```python
from build123d import *

# Parameters (mm, degrees)
CROQUIS1_R                 = 2
SALIENTE_EXTRUIR1_DEPTH    = 21
CORTAR_EXTRUIR1_DEPTH      = 43.09513036
CORTAR_EXTRUIR1_DEPTH_BACK = 5
CUT_EXTRUDE1_START         = 10
SKETCH2_R                  = 1.25
CUT_EXTRUDE1_DEPTH         = 3
LPATTERN1_COUNT            = 2
LPATTERN1_PITCH            = 20


with BuildPart() as part:
    # Croquis1 → Saliente-Extruir1 (new, symmetric)
    with BuildSketch(Plane(origin=(0, 0, 0), x_dir=(1, 0, 0), z_dir=(0, 1, 0))):
        with Locations(Location((0, 0, 0), (0, 0, 90))):
            Circle(CROQUIS1_R)
    extrude(amount=SALIENTE_EXTRUIR1_DEPTH, both=True)

    # Croquis2 → Cortar-Extruir1 (cut, two sides: drawn at the far end of the back side and taken through both)
    with BuildSketch(Plane(origin=(0, 21, 0), x_dir=(1, 0, 0), z_dir=(0, 1, 0)).offset(-CORTAR_EXTRUIR1_DEPTH_BACK)):
        Polygon((-21.233275663, 1.2), (-1.6, 1.2), (1.6, 1.2), (21.233275663, 1.2), (21.233275663, 40.466551326), (-21.233275663, 40.466551326), align=None)
    extrude(amount=CORTAR_EXTRUIR1_DEPTH + CORTAR_EXTRUIR1_DEPTH_BACK, mode=Mode.SUBTRACT)

    # Sketch2 → Cut-Extrude1 (cut)
    with BuildSketch(Plane(origin=(0, 0, 0), x_dir=(1, 0, 0), z_dir=(0, 1, 0)).offset(CUT_EXTRUDE1_START)):
        with Locations((2, 0)):
            Circle(SKETCH2_R)
    cut_extrude1 = extrude(amount=-CUT_EXTRUDE1_DEPTH, mode=Mode.SUBTRACT)

    # LPattern1: Cut-Extrude1 ×2
    with Locations(*[(0, -i * LPATTERN1_PITCH, 0) for i in range(1, LPATTERN1_COUNT)]):
        add(cut_extrude1, mode=Mode.SUBTRACT)


solid = part.part
```
Input: part model. Units: mm. Frame: model coordinates. A direction names the side the tool comes from. Give positions to 0.01 mm unless a question says otherwise; leave off trailing zeros. Write each loop counter-clockwise with the first axis right and the second up, starting at its lowest first coordinate (ties: lowest second). Pieces come first, ordered by that corner, then holes. Notation, with made-up numbers: (81.5, 16.25) - (131.5, 16.25) arc R20 ccw to (131.5, 36.25) - close; hole circle Ø4 at (78, -37). An arc over 180 degrees is marked (long way). Write item = value, one per line. Start each with the question number.
1. Mould query, pull axis Z, two halves, no side actions, for faces 1 (the cylindrical face through (-1.352, 0.294, 1.474)), 2 (the flat face through (0, 18, -1.2)), 3 (the cylindrical face through (0.75, -11.48, -0.02)). Classes: released by +Z, released by -Z, zero draft, split by the parting line, or undercut.
2. Section query D-D, the plane z = 1.6. Output: boundary loops of the cut face in (x, y).
3. First-contact query: pin 1 Ø1.5 at (y, z) = (-9, 1.5) entering from -X; pin 2 Ø1.5 at (x, y) = (-1, 6.5) entering from +Z. Flat tips, straight axial feed; report the tip coordinate or a pass-through.
4. Section query B-B, the plane y = -2.5. Output: boundary loops of the cut face in (x, z).
5. Section query C-C, the plane y = -12.5. Output: boundary loops of the cut face in (x, z), then the cut area to 3 significant figures.
6. Section query A-A, the plane z = 0. Output: boundary loops of the cut face in (x, y), then the cut area to 4 significant figures.
7. Ray query, L1, parallel to Y at x = 1.4, z = 0.3; L2, parallel to Z at x = -0.1, y = -10; L3, parallel to Z at x = -1.2, y = -19. Return the intervals inside material, ascending.
8. Access query for faces 4 (the flat face through (0, 16, -1.5)), 5 (the flat face through (1, -10, 0)), 6 (the flat face through (0, 21, 0)). Directions: +Z, -Z, +X, -X, +Y, -Y. A direction counts if a zero-diameter tool reaches every point of the face in a straight line with its end or side. Return the directions, or none.
Check sheet entries:
q1.face_1 = split by the parting line
q1.face_2 = released by -Z
q1.face_3 = undercut
q2.outline = (-1.2, -21) - (1.2, -21) - (1.2, 21) - (-1.2, 21) - close
q3.pin_1 = -1.85
q3.pin_2 = 1.98
q4.outline = circle Ø4 at (0, 0)
q5.outline = (1.61, -1.19) arc R1.25 cw to (1.61, 1.19) arc R2 ccw (long way) to start
q5.area = 10.4 mm2
q6.outline = (-2, -21) - (2, -21) - (2, -13) - (0.75, -13) - (0.75, -10) - (2, -10) - (2, 7) - (0.75, 7) - (0.75, 10) - (2, 10) - (2, 21) - (-2, 21) - close
q6.area = 160.5 mm2
q7.L1 = -21 to -13, -10 to 7, 10 to 21
q7.L2 = -2 to 2
q7.L3 = -1.6 to 1.6
q8.face_4 = -Z, +X, -X, +Y
q8.face_5 = +X
q8.face_6 = +Z, -Z, +X, -X, +Y
